from build123d import *

# Parameters (mm, degrees)
BOSS_EXTRUDE1_START = 9.525
SKETCH1_R           = 12
SKETCH1_R_2         = 1.7
SKETCH1_R_3         = 4
BOSS_EXTRUDE1_DEPTH = 2.12


with BuildPart() as part:
    # Sketch1 → Boss-Extrude1 (new body)
    with BuildSketch(Plane.XY.offset(BOSS_EXTRUDE1_START)):
        with Locations(Location((0, 0, 0), (0, 0, 270))):
            Circle(SKETCH1_R)
        with Locations(Location((-6.92820323, -4, 0), (0, 0, 270))):
            Circle(SKETCH1_R_2, mode=Mode.SUBTRACT)
        with Locations(Location((6.92820323, -4, 0), (0, 0, 270))):
            Circle(SKETCH1_R_2, mode=Mode.SUBTRACT)
        with Locations(Location((0, 8, 0), (0, 0, 270))):
            Circle(SKETCH1_R_2, mode=Mode.SUBTRACT)
        with Locations(Location((0, 0, 0), (0, 0, 270))):
            Circle(SKETCH1_R_3, mode=Mode.SUBTRACT)
    extrude(amount=BOSS_EXTRUDE1_DEPTH)


solid = part.part
Part model, mm, in its own coordinate system. Coordinates: 2 decimals unless noted, no trailing zeros. Loops run counter-clockwise (first coordinate to the right, second up) from the corner with the lowest first, then second, coordinate; pieces in that order, holes last. Notation, with made-up numbers: M 21.5,-33.5 L 72.5,-33.5 A17 ccw 72.5,-21.5 Z; hole C -1,67.5 d2. An arc over 180 degrees is marked long. Use a Markdown table: item, result. Add a question column.
Q1. Cut at C-C (x = 8.25). Write the cut outline in (y, z) (3 decimals), and give its area (3 significant figures).
Q2. Cut at B-B (x = -1). Write the cut outline in (y, z) (3 decimals).
Q3. Cut at A-A (y = 0). Write the cut outline in (x, z) (3 decimals).
Q4. Cut at D-D (y = -5.25). Write the cut outline in (x, z) (3 decimals), and give its area (3 significant figures).
Q5. Mould opens along Y. For faces 1 (the cylindrical face through (3.604, -11.446, 10.57)), 2 (the flat face through (3, 3, 9.525)), 3 (the cylindrical face through (6.28, -5.57, 10.57)) say: +Y half, -Y half, draft (parallel to the pull), parting line (faces both ways), or undercut.
Q6. Probe L1, parallel to X at y = 0, z = 10.3; L2, parallel to Y at x = 3, z = 11.2; L3, parallel to Y at x = 7.25, z = 11.55. List the from-to ranges inside material, lowest first.
Worked out:
| question | item | result |
|---|---|---|
| 1 | outline | M -8.714,9.525 L -5.069,9.525 L -5.069,11.645 L -8.714,11.645 Z; M -2.931,9.525 L 8.714,9.525 L 8.714,11.645 L -2.931,11.645 Z |
| 1 | area | 32.4 mm2 |
| 2 | outline | M -11.958,9.525 L -3.873,9.525 L -3.873,11.645 L -11.958,11.645 Z; M 3.873,9.525 L 6.625,9.525 L 6.625,11.645 L 3.873,11.645 Z; M 9.375,9.525 L 11.958,9.525 L 11.958,11.645 L 9.375,11.645 Z |
| 3 | outline | M -12,9.525 L -4,9.525 L -4,11.645 L -12,11.645 Z; M 4,9.525 L 12,9.525 L 12,11.645 L 4,11.645 Z |
| 4 | outline | M -10.791,9.525 L -8.08,9.525 L -8.08,11.645 L -10.791,11.645 Z; M -5.776,9.525 L 5.776,9.525 L 5.776,11.645 L -5.776,11.645 Z; M 8.08,9.525 L 10.791,9.525 L 10.791,11.645 L 8.08,11.645 Z |
| 4 | area | 36.0 mm2 |
| 5 | face 1 | parting line |
| 5 | face 2 | draft |
| 5 | face 3 | undercut |
| 6 | L1 | x = -12 to -4, 4 to 12 |
| 6 | L2 | y = -11.62 to -2.65, 2.65 to 11.62 |
| 6 | L3 | y = -9.56 to -5.67, -2.33 to 9.56 |
